Geometry check sheet. Reference: drawing and pictorial views, mm from the part's lowest x, y, z. A direction names the side the tool comes from. Round coordinates to 2 decimals unless told otherwise and drop trailing zeros. Order: outer loops, then holes, each group sorted by start corner. A loop starts at its lowest first (then second) coordinate and runs counter-clockwise, first axis right, second up.
(1) Sectioned sample at C-C (x = 66). Record the boundary of the cut face in (y, z), plus the area to 3 significant figures.
(2) Material ranges on line 1 along X through (y, z) = (5.5, 14.75); line 2 along Y through (x, z) = (60, 3.5); line 3 along Y through (x, z) = (60.5, 8.75), recorded low to high.
(3) Set-up check for the marked faces 1, 2 and 3: record each of +Z, -Z, +X, -X, +Y, -Y from which the full face is reachable in a straight line by a thin tool's end or side.
(4) Go/stop test with flat-tipped pins: pin 1 (5 mm diameter, centred on x = 9, z = 8, fed in from +Y); pin 2 (1.5 mm diameter, centred on x = 24.5, y = 14, fed in from +Z); pin 3 (2 mm diameter, centred on x = 16.5, y = 14.5, fed in from -Z). Record where each tip stops, or that it passes through.
(5) Sectioned sample at D-D (y = 2.25). Record the boundary of the cut face in (x, z), plus the area to 3 significant figures.
(6) Sectioned sample at A-A (z = 9). Record the boundary of the cut face in (x, y).
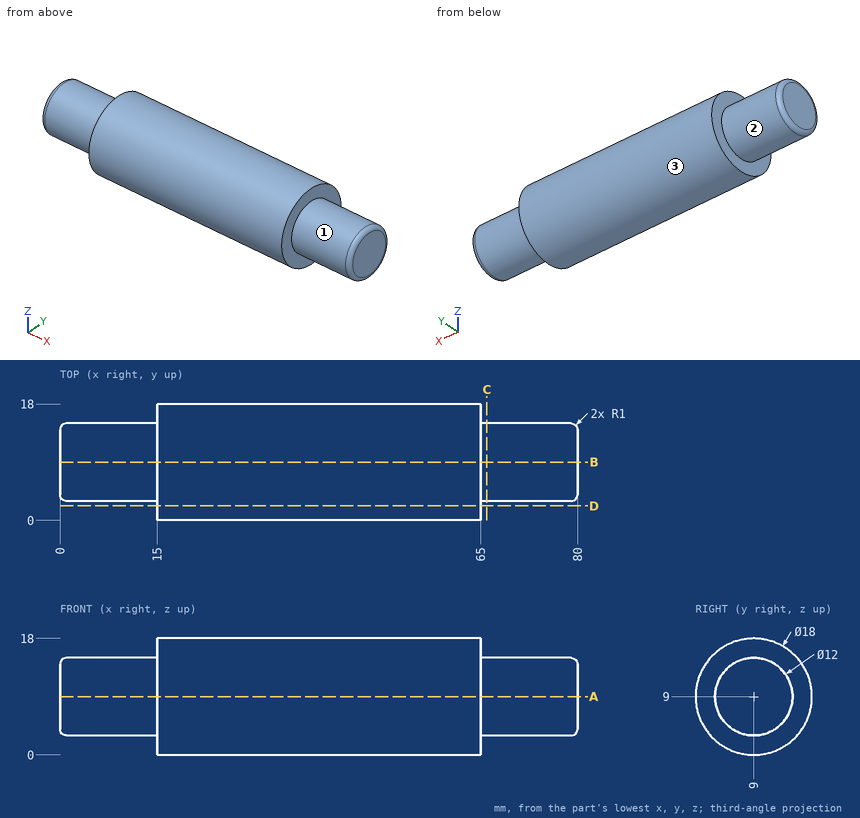
Answer below:
1. outline: circle Ø12 at (9, 9)
1. area: 113 mm2
2. line 1: x = 15 to 65
2. line 2: y = 1.88 to 16.12
2. line 3: y = 0 to 18
3. face 1: +X
3. face 2: -X
3. face 3: +X, -X
4. pin 1: stops at y = 15
4. pin 2: stops at z = 16.93
4. pin 3: stops at z = 1.21
5. outline: (15, 3.05) - (65, 3.05) - (65, 14.95) - (15, 14.95) - close
5. area: 595 mm2
6. outline: (0, 4) arc R1 ccw to (1, 3) - (15, 3) - (15, 0) - (65, 0) - (65, 3) - (79, 3) arc R1 ccw to (80, 4) - (80, 14) arc R1 ccw to (79, 15) - (65, 15) - (65, 18) - (15, 18) - (15, 15) - (1, 15) arc R1 ccw to (0, 14) - close
